The model under review builds one solid part; all positions refer to its coordinate system, in mm. A direction names the side the tool comes from. Round coordinates to 2 decimals unless told otherwise and drop trailing zeros. Loops run counter-clockwise (first coordinate to the right, second up) from the corner with the lowest first, then second, coordinate; pieces in that order, holes last. Notation, with made-up numbers: M 8.25,46 L 49.25,46 A28 cw 49.25,70 Z; hole C -37.75,82 d8. An arc over 180 degrees is marked long. One line per question, with ' | ' between items.
from build123d import *

# Parameters (mm, degrees)
CYLINDER004_R     = 6.5
CYLINDER004_DEPTH = 10
CYLINDER005_R     = 3.15
CYLINDER005_DEPTH = 10
BOX005_W          = 16
BOX005_H          = 9
BOX005_DEPTH      = 31
BOX004_W          = 28
BOX004_H          = 6
BOX004_DEPTH      = 30
CHAMFER017_SIZE   = 5
CHAMFER018_SIZE   = 2
CHAMFER019_SIZE   = 1
BOX006_W          = 7.8
BOX006_H          = 2
BOX006_DEPTH      = 30
CHAMFER008_SIZE   = 1


with BuildPart() as cylinder004:
    # Cylinder004 → Cylinder004 (new body)
    with BuildSketch(Plane(origin=(-15, -7, 15), x_dir=(1, 0, 0), z_dir=(0, 1, 0))):
        Circle(CYLINDER004_R)
    extrude(amount=CYLINDER004_DEPTH)


with BuildPart() as cylinder005:
    # Cylinder005 → Cylinder005 (new body)
    with BuildSketch(Plane(origin=(-15, 0, 15), x_dir=(1, 0, 0), z_dir=(0, 1, 0))):
        Circle(CYLINDER005_R)
    extrude(amount=CYLINDER005_DEPTH)


with BuildPart() as cube005:
    # Box005 → Box005 (new body)
    with BuildSketch(Plane(origin=(-7.5, 2.5, 0), x_dir=(1, 0, 0), z_dir=(0, 0, 1))):
        with Locations((8, 4.5)):
            Rectangle(BOX005_W, BOX005_H)
    extrude(amount=BOX005_DEPTH)


with BuildPart() as chamfer019:
    # Box004 → Box004 (new body)
    with BuildSketch(Plane(origin=(-28, 0, 0), x_dir=(1, 0, 0), z_dir=(0, 0, 1))):
        with Locations((14, 3)):
            Rectangle(BOX004_W, BOX004_H)
    extrude(amount=BOX004_DEPTH)

    # Cut002008006002: cut Cube005
    add(cube005.part, mode=Mode.SUBTRACT)

    # Chamfer017
    chamfer017_edges = [chamfer019.edges().sort_by_distance(p)[0] for p in [
        (0, 1.25, 30),
        (0, 1.25, 0),
    ]]
    chamfer(chamfer017_edges, length=CHAMFER017_SIZE)

    # Chamfer018
    chamfer018_edges = [chamfer019.edges().sort_by_distance(p)[0] for p in [
        (-28, 3, 0),
        (-28, 3, 30),
    ]]
    chamfer(chamfer018_edges, length=CHAMFER018_SIZE)

    # Chamfer019
    chamfer019_edges = [chamfer019.edges().sort_by_distance(p)[0] for p in [
        (-15.5, 0, 0),
        (-27, 0, 1),
        (-28, 0, 15),
        (-27, 0, 29),
        (-15.5, 0, 30),
        (-2.5, 0, 27.5),
        (0, 0, 15),
        (-2.5, 0, 2.5),
    ]]
    chamfer(chamfer019_edges, length=CHAMFER019_SIZE)


with BuildPart() as cut002008006004001:
    # Box006 → Box006 (new body)
    with BuildSketch(Plane(origin=(-18.9, 5, 0), x_dir=(1, 0, 0), z_dir=(0, 0, 1))):
        with Locations((3.9, 1)):
            Rectangle(BOX006_W, BOX006_H)
    extrude(amount=BOX006_DEPTH)

    # Chamfer008
    chamfer008_edges = [cut002008006004001.edges().sort_by_distance(p)[0] for p in [
        (-15, 7, 0),
        (-15, 7, 30),
    ]]
    chamfer(chamfer008_edges, length=CHAMFER008_SIZE)

    # Fusion009: union Chamfer019
    add(chamfer019.part)

    # Cut002008006003: cut Cylinder005
    add(cylinder005.part, mode=Mode.SUBTRACT)

    # Cut002008006004: cut Cylinder004
    add(cylinder004.part, mode=Mode.SUBTRACT)


solid = cut002008006004001.part
1) Add section C-C on y = 1.75. State the section outline as (x, z) points.
Output values:
outline: M -28,2 L -26,0 L -5,0 L 0,5 L 0,25 L -5,30 L -26,30 L -28,28 Z; hole C -15,15 d13
2) Add section A-A on x = -15. State the section outline as (y, z) points.
Output values:
outline: M 0,1 L 1,0 L 6,0 L 7,1 L 7,11.85 L 3,11.85 L 3,8.5 L 0,8.5 Z; M 0,21.5 L 3,21.5 L 3,18.15 L 7,18.15 L 7,29 L 6,30 L 1,30 L 0,29 Z
3) For line 1 (X direction, y = 1.3, z = 15); line 2 (Z direction, x = -15, y = 4); line 3 (Z direction, x = -15, y = 1.9), list the stretches that pass through material, from the lowest coordinate up.
Output values:
line 1: x = -28 to -21.5, -8.5 to 0 | line 2: z = 0 to 11.85, 18.15 to 30 | line 3: z = 0 to 8.5, 21.5 to 30
4) Insertion check: P1, Ø8, axis at x = -15, z = 15, coming from the -Y side; P2, Ø3, axis at x = -9.5, z = 20, coming from the +Y side; P3, Ø1.5, axis at x = -5, z = 14.5, coming from the +Y side. Each pin has a flat end and moves straight along its axis. Give the tip position at first contact, or say it passes through.
Output values:
P1: stops at y = 3 | P2: stops at y = 6 | P3: stops at y = 2.5
5) Add section D-D on z = 21. State the section outline as (x, y) points, then the cut area to 3 significant figures.
Output values:
outline: M -28,1 L -27,0 L -17.5,0 L -17.5,3 L -12.5,3 L -12.5,0 L -1,0 L 0,1 L 0,2.5 L -7.5,2.5 L -7.5,6 L -11.1,6 L -11.1,7 L -18.9,7 L -18.9,6 L -28,6 Z | area: 134 mm²
6) Machinability: for faces 1 (the flat face through (-8, 0, 15)), 2 (the flat face through (-11.1, 6.5, 14.8)), which of the approach directions +Z, -Z, +X, -X, +Y, -Y give a long, thin tool a straight path to every point of the face, cutting with its end or side? Answer none if there is none.
Output values:
face 1: +Z, -Z, +X, -X, -Y | face 2: +Z, -Z, +X, +Y
7) Add section B-B on z = 15. State the section outline as (x, y) points.
Output values:
outline: M -28,1 L -27,0 L -21.5,0 L -21.5,3 L -18.15,3 L -18.15,7 L -18.9,7 L -18.9,6 L -28,6 Z; M -11.85,3 L -8.5,3 L -8.5,0 L -1,0 L 0,1 L 0,2.5 L -7.5,2.5 L -7.5,6 L -11.1,6 L -11.1,7 L -11.85,7 Z
